Design review of the part built by this model. Coordinates are the model's own, in mm. Give positions to 0.01 mm unless a question says otherwise; leave off trailing zeros. Order: outer loops, then holes, each group sorted by start corner. A loop starts at its lowest first (then second) coordinate and runs counter-clockwise, first axis right, second up. Notation, with made-up numbers: M 89.25,25.25 L 93.25,25.25 A18 cw 93.25,29.25 Z; hole C 38,25.5 d6. An arc over 180 degrees is marked long. Answer as a JSON object with one key per item and string values.
from build123d import *

# Parameters (mm, degrees)
RESSALTO_EXTRUS_O1_DEPTH   = 3
ESBO_O2_W                  = 5.4
ESBO_O2_H                  = 3.1
CORTE_EXTRUS_O1_DEPTH      = 87.261231153
FURO_DE_DI_METRO_3_0_3_1_D = 3


with BuildPart() as part:
    # Esboço1 → Ressalto-extrusão1 (new body)
    with BuildSketch(Plane(origin=(0, 0, 0), x_dir=(1, 0, 0), z_dir=(0, 1, 0))):
        with BuildLine():
            Line((0, 4), (74.134848681, 4))
            ThreePointArc((74.134848681, 4), (75.296743684, 4.192654993), (76.334280425, 4.75))
            ThreePointArc((76.334280425, 4.75), (86, 0), (76.334280425, -4.75))
            ThreePointArc((76.334280425, -4.75), (75.296743684, -4.192654993), (74.134848681, -4))
            Line((74.134848681, -4), (0, -4))
            ThreePointArc((0, -4), (-4, 0), (0, 4))
        make_face()
    extrude(amount=-RESSALTO_EXTRUS_O1_DEPTH)

    # Esboço2 → Corte-extrusão1 (cut, through all)
    with BuildSketch(Plane(origin=(0, 0, 0), x_dir=(1, 0, 0), z_dir=(0, 1, 0))):
        with Locations((31, 0)):
            Rectangle(ESBO_O2_W, ESBO_O2_H)
    extrude(amount=-CORTE_EXTRUS_O1_DEPTH, mode=Mode.SUBTRACT)

    # Furo de diâmetro Ø3.0 (3)1 (through all)
    with Locations(Plane(origin=(0, 0, 0), x_dir=(1, 0, 0), z_dir=(0, 1, 0))):
        with Locations((0, 0), (80, 0)):
            Hole(FURO_DE_DI_METRO_3_0_3_1_D / 2)


solid = part.part
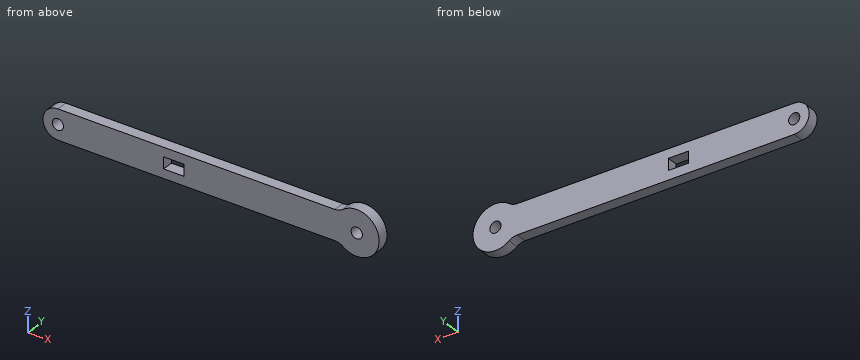
(1) We need section B-B (z = 0). Write out the cut boundary in (x, y), plus the area to 3 significant figures.
Checked values:
{"outline": "M -4,-3 L -1.5,-3 L -1.5,0 L -4,0 Z; M 1.5,-3 L 28.3,-3 L 28.3,0 L 1.5,0 Z; M 33.7,-3 L 78.5,-3 L 78.5,0 L 33.7,0 Z; M 81.5,-3 L 86,-3 L 86,0 L 81.5,0 Z", "area": "236 mm^2"}
(2) We need section A-A (x = 80). Write out the cut boundary in (y, z), plus the area to 3 significant figures.
Checked values:
{"outline": "M -3,-6 L 0,-6 L 0,-1.5 L -3,-1.5 Z; M -3,1.5 L 0,1.5 L 0,6 L -3,6 Z", "area": "27.0 mm^2"}
(3) We need section C-C (y = -2.2). Write out the cut boundary in (x, z), plus the area to 3 significant figures.
Checked values:
{"outline": "M 0,-4 L 74.13,-4 A3.6 cw 76.33,-4.75 A6 ccw long 76.33,4.75 A3.6 cw 74.13,4 L 0,4 A4 ccw Z; hole C 0,0 d3; hole M 28.3,-1.55 L 33.7,-1.55 L 33.7,1.55 L 28.3,1.55 Z; hole C 80,0 d3", "area": "704 mm^2"}
(4) To check wall thickness, follow L1, parallel to Z at x = 0, y = -1.35; L2, parallel to Z at x = 80, y = -1.3; L3, parallel to Z at x = 46, y = -1.85. State the ranges of each line that lie inside material, in increasing order. Write a range as from..to.
Checked values:
{"L1": "z = -4..-1.5, 1.5..4", "L2": "z = -6..-1.5, 1.5..6", "L3": "z = -4..4"}
(5) We need section D-D (x = 65). Write out the cut boundary in (y, z), plus the area to 3 significant figures.
Checked values:
{"outline": "M -3,-4 L 0,-4 L 0,4 L -3,4 Z", "area": "24.0 mm^2"}
(6) Insertion check: pin 1 (2.5 mm diameter, centred on x = 0, z = 0, fed in from -Y); pin 2 (5 mm diameter, centred on x = 35.5, z = -3, fed in from +Y); pin 3 (1.5 mm diameter, centred on y = -0.5, z = 1, fed in from +X); pin 4 (0.9 mm diameter, centred on x = 25.5, y = -1, fed in from +Z). Each pin has a flat end and moves straight along its axis. Give the tip position at first contact, or say it passes through.
Checked values:
{"pin 1": "passes through", "pin 2": "stops at y = 0", "pin 3": "stops at x = 85.99", "pin 4": "stops at z = 4"}
